```python
from build123d import *

# Parameters (mm, degrees)
SZKIC1_W                    = 54
SZKIC1_H                    = 71
DODANIE_WYCI_GNI_CIE1_DEPTH = 5
SZKIC2_W                    = 23.5
SZKIC2_H                    = 28
WYTNIJ_WYCI_GNI_CIE1_DEPTH  = 5
SZKIC3_W                    = 21
SZKIC3_H                    = 21
WYTNIJ_WYCI_GNI_CIE2_DEPTH  = 3
SZKIC4_R                    = 1.25
WYTNIJ_WYCI_GNI_CIE3_DEPTH  = 5
SZKIC5_W                    = 20
SZKIC5_H                    = 43
DODANIE_WYCI_GNI_CIE2_DEPTH = 5
SZKIC6_R                    = 8.5
WYTNIJ_WYCI_GNI_CIE4_DEPTH  = 5
SZKIC7_R                    = 3
WYTNIJ_WYCI_GNI_CIE5_DEPTH  = 10
ZAOKR_GLENIE3_R             = 10
SZKIC8_W                    = 19
SZKIC8_H                    = 28
DODANIE_WYCI_GNI_CIE3_DEPTH = 5
ZAOKR_GLENIE2_SIZE          = 2
SZKIC9_R                    = 2
WYTNIJ_WYCI_GNI_CIE6_DEPTH  = 10
SZKIC10_R                   = 1.5
WYTNIJ_WYCI_GNI_CIE7_DEPTH  = 10
ZAOKR_GLENIE4_R             = 2


with BuildPart() as part:
    # Szkic1 → Dodanie-wyciągnięcie1 (new body)
    with BuildSketch(Plane.XY):
        with Locations((7, 0.5)):
            Rectangle(SZKIC1_W, SZKIC1_H)
    extrude(amount=DODANIE_WYCI_GNI_CIE1_DEPTH)

    # Szkic2 → Wytnij-wyciągnięcie1 (cut)
    with BuildSketch(Plane.XY.offset(5)):
        with Locations((-8.25, 22)):
            Rectangle(SZKIC2_W, SZKIC2_H)
    extrude(amount=-WYTNIJ_WYCI_GNI_CIE1_DEPTH, mode=Mode.SUBTRACT)

    # Szkic3 → Wytnij-wyciągnięcie2 (cut)
    with BuildSketch(Plane(origin=(0, 0, 0), x_dir=(-1, 0, 0), z_dir=(0, 0, -1))):
        with Locations((-14, 20)):
            Rectangle(SZKIC3_W, SZKIC3_H)
    extrude(amount=-WYTNIJ_WYCI_GNI_CIE2_DEPTH, mode=Mode.SUBTRACT)

    # Szkic4 → Wytnij-wyciągnięcie3 (cut)
    with BuildSketch(Plane.XY.offset(5)):
        with Locations((6, 32.5)):
            Circle(SZKIC4_R)
        with Locations((14, 32.5)):
            Circle(SZKIC4_R)
        with Locations((22, 32.5)):
            Circle(SZKIC4_R)
        with Locations((22, 5.5)):
            Circle(SZKIC4_R)
        with Locations((6, 5.5)):
            Circle(SZKIC4_R)
        with Locations((27.5, 27)):
            Circle(SZKIC4_R)
        with Locations((27.5, 11)):
            Circle(SZKIC4_R)
    extrude(amount=-WYTNIJ_WYCI_GNI_CIE3_DEPTH, mode=Mode.SUBTRACT)

    # Szkic5 → Dodanie-wyciągnięcie2 (add)
    with BuildSketch(Plane.XY.offset(5)):
        with Locations((-30, -13.5)):
            Rectangle(SZKIC5_W, SZKIC5_H)
    extrude(amount=-DODANIE_WYCI_GNI_CIE2_DEPTH)

    # Szkic6 → Wytnij-wyciągnięcie4 (cut)
    with BuildSketch(Plane.XY.offset(5)):
        with Locations((-20, -4)):
            Circle(SZKIC6_R)
        with Locations((14, -4)):
            Circle(SZKIC6_R)
    extrude(amount=-WYTNIJ_WYCI_GNI_CIE4_DEPTH, mode=Mode.SUBTRACT)

    # Szkic7 → Wytnij-wyciągnięcie5 (cut)
    with BuildSketch(Plane.XY.offset(5)):
        with Locations((-11, -30)):
            Circle(SZKIC7_R)
        with Locations((5, -30)):
            Circle(SZKIC7_R)
        with Locations((-35, -19)):
            Circle(SZKIC7_R)
        with Locations((29, -19)):
            Circle(SZKIC7_R)
    extrude(amount=-WYTNIJ_WYCI_GNI_CIE5_DEPTH, mode=Mode.SUBTRACT)

    # Zaokrąglenie3
    zaokr_glenie3_edges = [part.edges().sort_by_distance(p)[0] for p in [
        (-40, -35, 2.5),
        (34, -35, 2.5),
    ]]
    fillet(zaokr_glenie3_edges, radius=ZAOKR_GLENIE3_R)

    # Szkic8 → Dodanie-wyciągnięcie3 (add)
    with BuildSketch(Plane.XY.offset(5)):
        with Locations((-30.5, 22)):
            Rectangle(SZKIC8_W, SZKIC8_H)
    extrude(amount=-DODANIE_WYCI_GNI_CIE3_DEPTH)

    # Zaokrąglenie2
    # a fillet whose section is not a circle: 2 mm, written as the material it adds along each edge
    with BuildSketch(Plane(origin=(3.5, 8, 5), x_dir=(0, 1, 0), z_dir=(0, 0, -1))) as zaokr_glenie2_piece_1_section:
        with BuildLine():
            Bezier((ZAOKR_GLENIE2_SIZE, 0), (0, 0), (0, -ZAOKR_GLENIE2_SIZE), weights=[1, 1, 1])
            Line((0, -ZAOKR_GLENIE2_SIZE), (0, 0))
            Line((0, 0), (ZAOKR_GLENIE2_SIZE, 0))
        make_face()
    zaokr_glenie2_piece_1 = extrude(amount=5, mode=Mode.PRIVATE)
    zaokr_glenie2_piece_1 = split(zaokr_glenie2_piece_1, bisect_by=Plane(origin=(3.5, 9.5, 5), z_dir=(0, 1, 0)), keep=Keep.TOP, mode=Mode.PRIVATE)
    zaokr_glenie2_piece_1 = split(zaokr_glenie2_piece_1, bisect_by=Plane(origin=(3.5, 8, 3), z_dir=(0, 0, 1)), keep=Keep.TOP, mode=Mode.PRIVATE)
    add(zaokr_glenie2_piece_1)
    with BuildSketch(Plane(origin=(3.5, 8, 5), x_dir=(0, 1, 0), z_dir=(0, 0, -1))) as zaokr_glenie2_piece_2_section:
        with BuildLine():
            Bezier((ZAOKR_GLENIE2_SIZE, 0), (0, 0), (0, -ZAOKR_GLENIE2_SIZE), weights=[1, 1, 1])
            Line((0, -ZAOKR_GLENIE2_SIZE), (0, 0))
            Line((0, 0), (ZAOKR_GLENIE2_SIZE, 0))
        make_face()
    zaokr_glenie2_piece_2 = extrude(amount=5, mode=Mode.PRIVATE)
    zaokr_glenie2_piece_2 = split(zaokr_glenie2_piece_2, bisect_by=Plane(origin=(3.5, 9.5, 5), z_dir=(0, -1, 0)), keep=Keep.TOP, mode=Mode.PRIVATE)
    zaokr_glenie2_piece_2 = split(zaokr_glenie2_piece_2, bisect_by=Plane(origin=(3.5, 8, 3), z_dir=(0, 0, 1)), keep=Keep.TOP, mode=Mode.PRIVATE)
    add(zaokr_glenie2_piece_2)
    with BuildSketch(Plane(origin=(3.5, 8, 5), x_dir=(0, 1, 0), z_dir=(0, 0, -1))) as zaokr_glenie2_piece_3_section:
        with BuildLine():
            Bezier((ZAOKR_GLENIE2_SIZE, 0), (0, 0), (0, -ZAOKR_GLENIE2_SIZE), weights=[1, 1, 1])
            Line((0, -ZAOKR_GLENIE2_SIZE), (0, 0))
            Line((0, 0), (ZAOKR_GLENIE2_SIZE, 0))
        make_face()
    zaokr_glenie2_piece_3 = extrude(amount=5, mode=Mode.PRIVATE)
    zaokr_glenie2_piece_3 = split(zaokr_glenie2_piece_3, bisect_by=Plane(origin=(3.5, 9.5, 5), z_dir=(0, -1, 0)), keep=Keep.TOP, mode=Mode.PRIVATE)
    zaokr_glenie2_piece_3 = split(zaokr_glenie2_piece_3, bisect_by=Plane(origin=(3.5, 8, 3), z_dir=(0, 0, -1)), keep=Keep.TOP, mode=Mode.PRIVATE)
    add(zaokr_glenie2_piece_3)
    with BuildSketch(Plane(origin=(-21, 8, 5), x_dir=(1, 0, 0), z_dir=(0, 0, -1))) as zaokr_glenie2_piece_4:
        with BuildLine():
            Bezier((ZAOKR_GLENIE2_SIZE, 0), (0, 0), (0, -ZAOKR_GLENIE2_SIZE), weights=[1, 1, 1])
            Line((0, -ZAOKR_GLENIE2_SIZE), (0, 0))
            Line((0, 0), (ZAOKR_GLENIE2_SIZE, 0))
        make_face()
    extrude(amount=5)

    # Szkic9 → Wytnij-wyciągnięcie6 (cut)
    with BuildSketch(Plane.XY.offset(5)):
        with Locations((-27, 31)):
            Circle(SZKIC9_R)
        with Locations((-27, 21)):
            Circle(SZKIC9_R)
    extrude(amount=-WYTNIJ_WYCI_GNI_CIE6_DEPTH, mode=Mode.SUBTRACT)

    # Szkic10 → Wytnij-wyciągnięcie7 (cut)
    with BuildSketch(Plane.XY.offset(5)):
        with Locations((-3, -21)):
            Circle(SZKIC10_R)
    extrude(amount=-WYTNIJ_WYCI_GNI_CIE7_DEPTH, mode=Mode.SUBTRACT)

    # Zaokrąglenie4
    zaokr_glenie4_edges = [part.edges().sort_by_distance(p)[0] for p in [
        (24.5, 9.5, 1.5),
        (24.5, 30.5, 1.5),
    ]]
    fillet(zaokr_glenie4_edges, radius=ZAOKR_GLENIE4_R)


solid = part.part
```
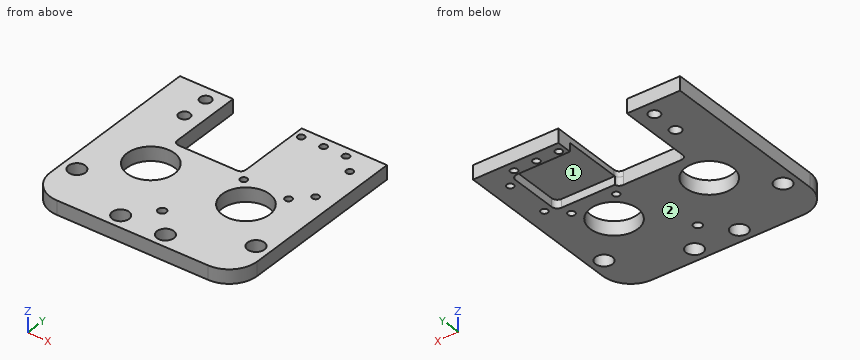
The listing builds one solid part. Answer for the finished solid, in the listing's coordinates (mm). Face numbers are marked on the shaded views. Give positions to 0.01 mm unless a question says otherwise; leave off trailing zeros. Order: outer loops, then holes, each group sorted by start corner. A loop starts at its lowest first (then second) coordinate and runs counter-clockwise, first axis right, second up. Notation, with made-up numbers: (72, -19) -> (127, -19) arc R18 ccw to (127, 5) -> close; hole circle Ø5 at (19, 24). An arc over 180 degrees is marked (long way). Answer as CSV lines item,"result". Start each with the question number.
Q1. A cutting plane is placed at C-C (y = -21). Determine the outline of the cut face in (x, z).
Q2. Given pin 1 (1.5 mm diameter, centred on x = 22, y = 5.5, fed in from -Z); pin 2 (1.5 mm diameter, centred on x = -9.5, z = 2.5, fed in from +Y), each flat-ended and moving along its own axis, determine where each tip first touches the part or whether it passes through.
Q3. Find the intervals of material crossed by L1, parallel to Y at x = 14, z = 2.95; L2, parallel to Y at x = -3, z = 1.85; L3, parallel to X at y = 15, z = 4.75, in increasing order.
Q4. A cutting plane is placed at B-B (y = 15.5). Determine the outline of the cut face in (x, z), then the cut area to 4 significant figures.
Q5. A cutting plane is placed at D-D (z = 1.8). Count the separate pieces of the cut face and the enclosed holes in it, then the cut area to 3 significant figures.
Q6. Determine the mould class of the marked faces 1 and 2 for opening direction X: pulls with the +X half, pulls with the -X half, needs draft (parallel to the pull), parting line crosses it, or undercut.
Q7. A cutting plane is placed at A-A (x = 14). Determine the outline of the cut face in (y, z).
Results found:
1,outline,"(-40, 0) -> (-37.24, 0) -> (-37.24, 5) -> (-40, 5) -> close; (-32.76, 0) -> (-4.5, 0) -> (-4.5, 5) -> (-32.76, 5) -> close; (-1.5, 0) -> (26.76, 0) -> (26.76, 5) -> (-1.5, 5) -> close; (31.24, 0) -> (34, 0) -> (34, 5) -> (31.24, 5) -> close"
2,pin 1,"through"
2,pin 2,"y = 8"
3,L1,"-35 to -12.5, 4.5 to 9.5, 30.5 to 31.25, 33.75 to 36"
3,L2,"-35 to -22.5, -19.5 to 8"
3,L3,"-40 to -21, 3.5 to 34"
4,outline,"(-40, 0) -> (-21, 0) -> (-21, 5) -> (-40, 5) -> close; (3.5, 3) -> (24.5, 3) -> (24.5, 0) -> (34, 0) -> (34, 5) -> (3.5, 5) -> close"
4,area,"184.5 mm2"
5,separate pieces,"1"
5,enclosed holes,"16"
5,area,"3,450 mm2"
6,face 1,"undercut"
6,face 2,"needs draft"
7,outline,"(-35, 0) -> (-12.5, 0) -> (-12.5, 5) -> (-35, 5) -> close; (4.5, 0) -> (9.5, 0) -> (9.5, 3) -> (30.5, 3) -> (30.5, 0) -> (31.25, 0) -> (31.25, 5) -> (4.5, 5) -> close; (33.75, 0) -> (36, 0) -> (36, 5) -> (33.75, 5) -> close"
